Source: CAD feature listing. Evaluate the final solid. Frame: model axes, mm. Round coordinates to 2 decimals unless told otherwise and drop trailing zeros. Loops run counter-clockwise (first coordinate to the right, second up) from the corner with the lowest first, then second, coordinate; pieces in that order, holes last. Notation, with made-up numbers: (38, -28.5) - (52, -28.5) arc R16 cw to (52, 2.5) - close; hole circle Ø8 at (85.25, 43.5). An arc over 180 degrees is marked (long way). Write item = value, one per line. Start each with the question number.
from build123d import *

# Parameters (mm, degrees)
CYLINDER178_R     = 1.5
CYLINDER178_DEPTH = 55
CYLINDER172_R     = 3.5
CYLINDER172_DEPTH = 6.6


with BuildPart() as cylinder178:
    # Cylinder178 → Cylinder178 (new body)
    with BuildSketch(Plane(origin=(92.7, 68.9, 48.1), x_dir=(0, 0, -1), z_dir=(1, 0, 0))):
        Circle(CYLINDER178_R)
    extrude(amount=CYLINDER178_DEPTH)


with BuildPart() as cut210:
    # Cylinder172 → Cylinder172 (new body)
    with BuildSketch(Plane(origin=(99.1, 68.9, 48.1), x_dir=(0, 0, -1), z_dir=(1, 0, 0))):
        Circle(CYLINDER172_R)
    extrude(amount=CYLINDER172_DEPTH)

    # Cut210: cut Cylinder178
    add(cylinder178.part, mode=Mode.SUBTRACT)


solid = cut210.part
(1) Cut plane A-A (z = 48.1). Output: boundary loops of the cut face in (x, y), and give its area (3 significant figures).
(2) Cut plane C-C (x = 101.75). Output: boundary loops of the cut face in (y, z).
(3) Cut plane B-B (y = 69). Output: boundary loops of the cut face in (x, z).
(4) Pin query (flat end, axial travel): P1, Ø3, axis at x = 101.5, z = 45.5, coming from the +Y side; P2, Ø2, axis at x = 100, z = 48.5, coming from the +Y side; P3, Ø2.5, axis at y = 68.9, z = 48.1, coming from the -X side. Return the tip coordinate at first contact, or that it passes through.
(5) Mould query, pull axis Z, two halves, no side actions, for faces 1 (the face through (102.354, 65.795, 46.485)), 2 (the face through (105.7, 67, 48)), 3 (the face through (102.354, 70.165, 47.294)). Classes: +Z half, -Z half, draft (parallel to the pull), parting line (faces both ways), or undercut.
(6) Material intervals for line 1 along Y through (x, z) = (102, 48.1); line 2 along Z through (x, y) = (101, 67.75); line 3 along Y through (x, z) = (105.25, 46.75), sorted ascending. Write a range as from..to.
(7) Cut plane D-D (y = 70.75). Output: boundary loops of the cut face in (x, z), and give its area (3 significant figures).
Solution:
q1.outline = (99.1, 65.4) - (105.7, 65.4) - (105.7, 67.4) - (99.1, 67.4) - close; (99.1, 70.4) - (105.7, 70.4) - (105.7, 72.4) - (99.1, 72.4) - close
q1.area = 26.4 mm^2
q2.outline = circle Ø7 at (68.9, 48.1); hole circle Ø3 at (68.9, 48.1)
q3.outline = (99.1, 44.6) - (105.7, 44.6) - (105.7, 46.6) - (99.1, 46.6) - close; (99.1, 49.6) - (105.7, 49.6) - (105.7, 51.6) - (99.1, 51.6) - close
q4.P1 = 72.22
q4.P2 = 72.4
q4.P3 = through
q5.face_1 = parting line
q5.face_2 = draft
q5.face_3 = undercut
q6.line_1 = 65.4..67.4, 70.4..72.4
q6.line_2 = 44.79..47.14, 49.06..51.41
q6.line_3 = 65.67..68.25, 69.55..72.13
q7.outline = (99.1, 45.13) - (105.7, 45.13) - (105.7, 51.07) - (99.1, 51.07) - close
q7.area = 39.2 mm^2
